from build123d import *

# Parameters (mm, degrees)
PAD_DEPTH         = 6
SKETCH001_W       = 4
SKETCH001_H       = 6
PAD001_DEPTH      = 25.4
SKETCH002_R       = 1.5
POCKET_DEPTH      = 100
POCKET_DEPTH_BACK = 100
SKETCH003_W       = 35
SKETCH003_H       = 5
PAD002_DEPTH      = 15
SKETCH012_W       = 5.5
SKETCH012_H       = 5.5
SKETCH012_R       = 1.5
PAD010_DEPTH      = 26


with BuildPart() as part:
    # Sketch → Pad (new body)
    with BuildSketch(Plane.YZ):
        Polygon((-61.51, 65.6), (61.49, 65.6), (61.49, -9.4), (48.98, -19.508726), (-49, -19.508726), (-61.51, -9.4), align=None)
    extrude(amount=PAD_DEPTH)

    # Sketch001 (on Face8 of Pad) → Pad001 (join)
    with BuildSketch(Plane.YZ.offset(6)):
        with Locations((34.974674, 19.94)):
            Rectangle(SKETCH001_W, SKETCH001_H)
        with Locations((58.474674, 19.94)):
            Rectangle(SKETCH001_W, SKETCH001_H)
        with Locations((-34.517246, 19.94)):
            Rectangle(SKETCH001_W, SKETCH001_H)
        with Locations((-58.017246, 19.94)):
            Rectangle(SKETCH001_W, SKETCH001_H)
    extrude(amount=PAD001_DEPTH)

    # Sketch002 (on Face14 of Pad001) → Pocket (cut, two sides)
    with BuildSketch(Plane(origin=(0, 32.974674, 0), x_dir=(0, 0, -1), z_dir=(0, -1, 0))) as pocket_sk:
        with Locations((-20.1, 26.2)):
            Circle(SKETCH002_R)
        with Locations((-20.1, 8.2)):
            Circle(SKETCH002_R)
    extrude(amount=-POCKET_DEPTH, mode=Mode.SUBTRACT)
    extrude(pocket_sk.sketch, amount=POCKET_DEPTH_BACK, mode=Mode.SUBTRACT)

    # Sketch003 (on Face5 of Pocket) → Pad002 (join)
    with BuildSketch(Plane.YZ.offset(6)):
        with Locations((1.141409, -16.950097)):
            Rectangle(SKETCH003_W, SKETCH003_H)
    extrude(amount=PAD002_DEPTH)

    # Sketch012 (on Face5 of Pad002) → Pad010 (join)
    with BuildSketch(Plane.YZ.offset(6)):
        with Locations((-31.36108, 43.961174)):
            Rectangle(SKETCH012_W, SKETCH012_H)
        with Locations((-31.36108, 43.961174)):
            Circle(SKETCH012_R, mode=Mode.SUBTRACT)
        with Locations((32.670517, -12.15361)):
            Rectangle(SKETCH012_W, SKETCH012_H)
        with Locations((32.670517, -12.15361)):
            Circle(SKETCH012_R, mode=Mode.SUBTRACT)
    extrude(amount=PAD010_DEPTH)


solid = part.part
Verification items for the finished model (mm, model axes). A direction names the side the tool comes from. Give positions to 0.01 mm unless a question says otherwise; leave off trailing zeros. Write each loop counter-clockwise with the first axis right and the second up, starting at its lowest first coordinate (ties: lowest second). Pieces come first, ordered by that corner, then holes. Notation, with made-up numbers: (75.25, -20) - (119.25, -20) arc R25 ccw to (119.25, 19) - close; hole circle Ø8 at (54.25, 75). An arc over 180 degrees is marked (long way). Answer as CSV lines item,"result". Start each with the question number.
1. Depth check by flat-ended pin: pin 1 (1.5 mm diameter, centred on y = 32.5, z = -11.5, fed in from +X); pin 2 (1.8 mm diameter, centred on x = 16.5, z = 19, fed in from -Y); pin 3 (2 mm diameter, centred on y = -33.5, z = 21, fed in from +X). Enter the tip coordinate at first touch or a pass-through.
2. Sectioned sample at A-A (x = 11.5). Count the separate pieces of the cut face and the enclosed holes in it, then the cut area to 3 significant figures.
3. Set-up check for faces 4 (the face through (19, -35, 22.94)), 5 (the face through (19, 36.975, 20)), 6 (the face through (19, -34.111, 44)): record each of +Z, -Z, +X, -X, +Y, -Y from which the full face is reachable in a straight line by a thin tool's end or side.
4. Sectioned sample at D-D (x = 23). Record the boundary of the cut face in (y, z), then the cut area to 3 significant figures.
5. Sectioned sample at C-C (y = 9). Record the boundary of the cut face in (x, z), then the cut area to 3 significant figures.
6. Draft check along Y on faces 1 (the face through (19, -56.017, 20)), 2 (the face through (3, 55.3, -14.4)), 3 (the face through (19, -31, 46.711)). Enter one of: pulls with the +Y half, pulls with the -Y half, needs draft (parallel to the pull), parting line crosses it, or undercut.
7. Thickness scan on line 1 (X direction, y = 59.2, z = 20.1); line 2 (Z direction, x = 8, y = -35); line 3 (X direction, y = 10.5, z = 24). Record the ranges inside material, lowest first.
Derived:
1,pin 1,"x = 6"
1,pin 2,"y = -60.02"
1,pin 3,"x = 31.4"
2,separate pieces,"7"
2,enclosed holes,"2"
2,area,"317 mm²"
3,face 4,"+X, +Y, -Y"
3,face 5,"+Z, -Z, +X"
3,face 6,"+Z, +X, -Y"
4,outline,"(-60.02, 16.94) - (-56.02, 16.94) - (-56.02, 22.94) - (-60.02, 22.94) - close; (-36.52, 16.94) - (-32.52, 16.94) - (-32.52, 22.94) - (-36.52, 22.94) - close; (-34.11, 41.21) - (-28.61, 41.21) - (-28.61, 46.71) - (-34.11, 46.71) - close; (29.92, -14.9) - (35.42, -14.9) - (35.42, -9.4) - (29.92, -9.4) - close; (32.97, 16.94) - (36.97, 16.94) - (36.97, 22.94) - (32.97, 22.94) - close; (56.47, 16.94) - (60.47, 16.94) - (60.47, 22.94) - (56.47, 22.94) - close; hole circle Ø3 at (-31.36, 43.96); hole circle Ø3 at (32.67, -12.15)"
4,area,"142 mm²"
5,outline,"(0, -19.51) - (6, -19.51) - (6, -19.45) - (21, -19.45) - (21, -14.45) - (6, -14.45) - (6, 65.6) - (0, 65.6) - close"
5,area,"586 mm²"
6,face 1,"undercut"
6,face 2,"pulls with the +Y half"
6,face 3,"needs draft"
7,line 1,"0 to 6.7, 9.7 to 24.7, 27.7 to 31.4"
7,line 2,"16.94 to 18.61, 21.59 to 22.94"
7,line 3,"0 to 6"
